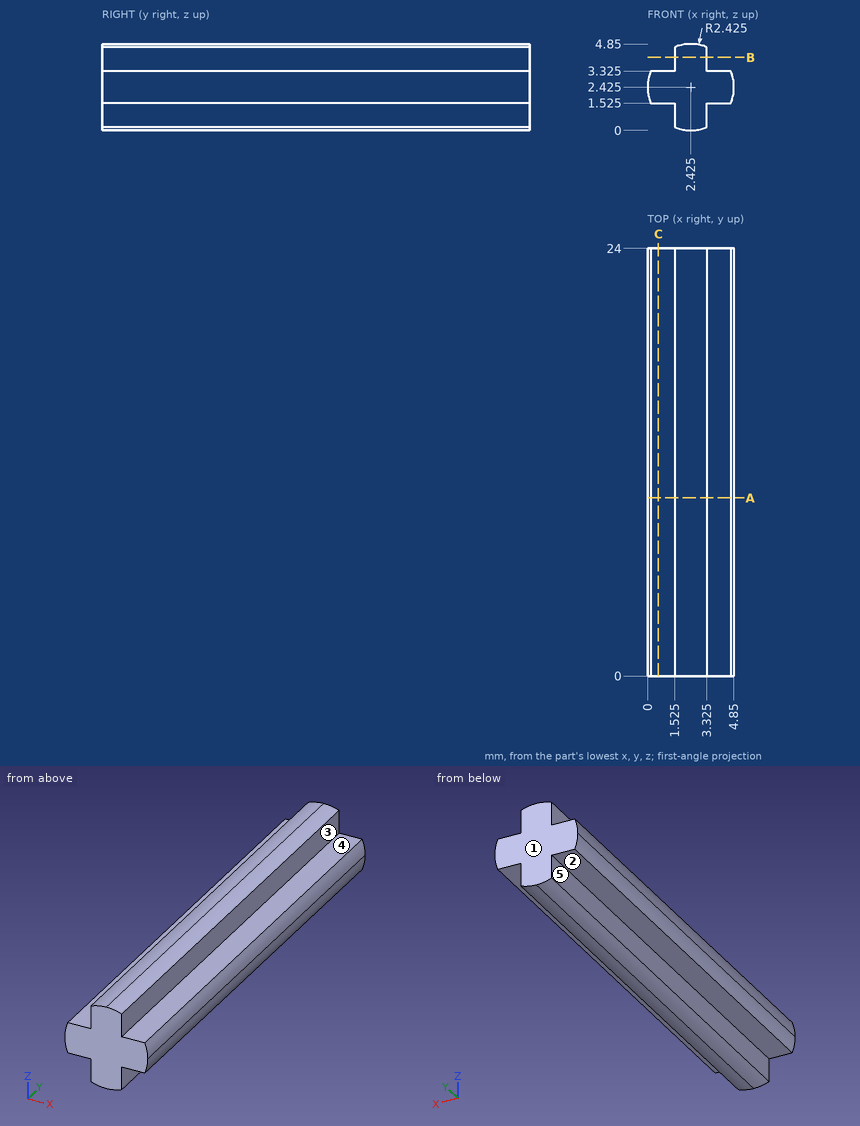
Check sheet for the drawn part. Datum: minimum x, y, z corner. Units: mm. A direction names the side the tool comes from. Round coordinates to 2 decimals unless told otherwise and drop trailing zeros. Order: outer loops, then holes, each group sorted by start corner. A loop starts at its lowest first (then second) coordinate and runs counter-clockwise, first axis right, second up.
(1) Access from +Z, -Z, +X, -X, +Y, -Y to the whole of each face (thin tool, end or side, straight path). Record for the marked faces 1 and 2.
(2) Draft check along X on the marked faces 3, 4 and 5. Enter one of: pulls with the +X half, pulls with the -X half, needs draft (parallel to the pull), parting line crosses it, or undercut.
(3) Cross-section at C-C, the plane x = 0.6. Enter the section's corners in (y, z) (3 decimals).
(4) Cross-section at B-B, the plane z = 4.1. Enter the section's corners in (x, y) (3 decimals).
(5) Go/stop test with flat-tipped pins: P1, Ø1.1, axis at y = 9.5, z = 4, coming from the +X side (3 decimals); P2, Ø1.1, axis at x = 4, y = 13, coming from the -Z side (3 decimals); P3, Ø1.5, axis at y = 12.5, z = 1, coming from the +X side. Record where each tip stops, or that it passes through.
(6) Scan lines: probe 1 along Z at (x, y) = (3.55, 10.5) (3 decimals); probe 2 along Z at (x, y) = (2.05, 6.5). Record each from-to range of solid material in increasing order.
(7) Cross-section at A-A, the plane y = 10. Enter the section's corners in (x, z) (3 decimals), and give its area (3 significant figures).
Check sheet entries:
1. face 1: +Z, -Z, +X, -X, +Y
1. face 2: -Z, -X, +Y, -Y
2. face 3: pulls with the +X half
2. face 4: needs draft
2. face 5: pulls with the -X half
3. outline: (0, 1.525) - (24, 1.525) - (24, 3.325) - (0, 3.325) - close
4. outline: (1.525, 0) - (3.325, 0) - (3.325, 24) - (1.525, 24) - close
5. P1: stops at x = 3.325
5. P2: stops at z = 1.525
5. P3: stops at x = 4.75
6. probe 1: z = 1.525 to 3.325
6. probe 2: z = 0.03 to 4.82
7. outline: (0, 2.425) arc R2.425 ccw to (0.173, 1.525) - (1.525, 1.525) - (1.525, 0.173) arc R2.425 ccw to (2.425, 0) arc R2.425 ccw to (3.325, 0.173) - (3.325, 1.525) - (4.677, 1.525) arc R2.425 ccw to (4.85, 2.425) arc R2.425 ccw to (4.677, 3.325) - (3.325, 3.325) - (3.325, 4.677) arc R2.425 ccw to (2.425, 4.85) arc R2.425 ccw to (1.525, 4.677) - (1.525, 3.325) - (0.173, 3.325) arc R2.425 ccw to start
7. area: 13.8 mm2
